from build123d import *

# Parameters (mm, degrees)
SKETCH1_R           = 12.35
BOSS_EXTRUDE1_DEPTH = 68
SKETCH2_R           = 3.55
BOSS_EXTRUDE2_DEPTH = 3
SKETCH3_R           = 2
BOSS_EXTRUDE3_DEPTH = 9.7
SKETCH5_W           = 12.75
SKETCH5_H           = 3
BOSS_EXTRUDE4_DEPTH = 14
SKETCH4_R           = 1.5
CUT_EXTRUDE1_DEPTH  = 3


with BuildPart() as part:
    # Sketch1 → Boss-Extrude1 (new body)
    with BuildSketch(Plane(origin=(0, 0, 0), x_dir=(1, 0, 0), z_dir=(0, 1, 0))):
        Circle(SKETCH1_R)
    extrude(amount=BOSS_EXTRUDE1_DEPTH)

    # Sketch2 → Boss-Extrude2 (add)
    with BuildSketch(Plane(origin=(0, 68, 0), x_dir=(1, 0, 0), z_dir=(0, 1, 0))):
        Circle(SKETCH2_R)
    extrude(amount=BOSS_EXTRUDE2_DEPTH)

    # Sketch3 → Boss-Extrude3 (add)
    with BuildSketch(Plane(origin=(0, 71, 0), x_dir=(1, 0, 0), z_dir=(0, 1, 0))):
        Circle(SKETCH3_R)
    extrude(amount=BOSS_EXTRUDE3_DEPTH)

    # Sketch5 → Boss-Extrude4 (add)
    with BuildSketch(Plane(origin=(0, 0, 0), x_dir=(0, 0, -1), z_dir=(1, 0, 0))):
        with Locations((0, 11.5)):
            Rectangle(SKETCH5_W, SKETCH5_H)
    extrude(amount=BOSS_EXTRUDE4_DEPTH)

    # Sketch4 → Cut-Extrude1 (cut)
    with BuildSketch(Plane(origin=(0, 68, 0), x_dir=(1, 0, 0), z_dir=(0, 1, 0))):
        with Locations((0, 8.5)):
            Circle(SKETCH4_R)
        with Locations((0, -8.5)):
            Circle(SKETCH4_R)
    extrude(amount=-CUT_EXTRUDE1_DEPTH, mode=Mode.SUBTRACT)


solid = part.part
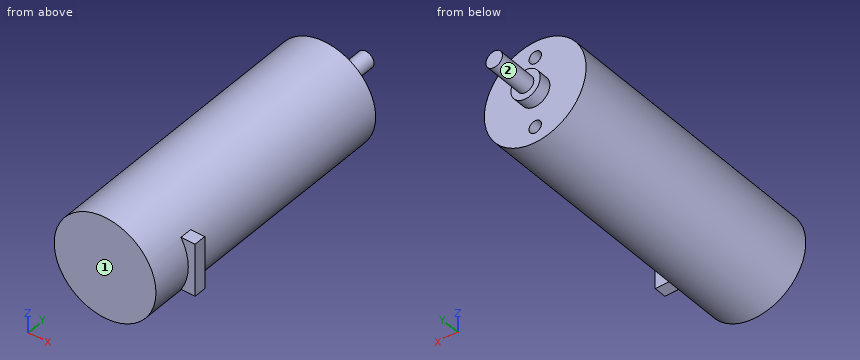
Source: CAD feature listing. Evaluate the final solid. Frame: model axes, mm. Face numbers are marked on the shaded views. A direction names the side the tool comes from. Give positions to 0.01 mm unless a question says otherwise; leave off trailing zeros. Write each loop counter-clockwise with the first axis right and the second up, starting at its lowest first coordinate (ties: lowest second). Pieces come first, ordered by that corner, then holes. Notation, with made-up numbers: (41.25, -34) - (85.25, -34) arc R31 cw to (85.25, -3) - close; hole circle Ø11 at (15.5, -36.5). An arc over 180 degrees is marked (long way). Write item = value, one per line. Start each with the question number.
Q1. Cut plane B-B, the plane z = 0. Return loops of the section in (x, y).
Q2. Reachability of the marked faces 1 and 2 from +Z, -Z, +X, -X, +Y, -Y: full face, straight path, thin tool, end or side. Return the list, or none.
Q3. Cut plane C-C, the plane y = 72. Return loops of the section in (x, z).
Q4. Material intervals for probe 1 along Z at (x, y) = (0, 66); probe 2 along Z at (x, y) = (7.25, 38.5); probe 3 along Y at (x, z) = (5, -7), sorted ascending.
Q5. Pin query (flat end, axial travel): pin 1 Ø2.5 at (x, y) = (12.5, 12) entering from +Z (3 decimals); pin 2 Ø1.5 at (y, z) = (67.5, -4) entering from +X; pin 3 Ø0.9 at (x, y) = (12, 11.5) entering from -Z (3 decimals). Return the tip coordinate at first contact, or that it passes through.
Q6. Cut plane D-D, the plane z = -8.5. Return loops of the section in (x, y), then the cut area to 3 significant figures.
Q7. Cut plane A-A, the plane x = 0. Return loops of the section in (y, z), then the cut area to 3 significant figures.
Computed values:
q1.outline = (-12.35, 0) - (12.35, 0) - (12.35, 10) - (14, 10) - (14, 13) - (12.35, 13) - (12.35, 68) - (3.55, 68) - (3.55, 71) - (2, 71) - (2, 80.7) - (-2, 80.7) - (-2, 71) - (-3.55, 71) - (-3.55, 68) - (-12.35, 68) - close
q2.face_1 = +Z, -Z, +X, -X, -Y
q2.face_2 = +Y
q3.outline = circle Ø4 at (0, 0)
q4.probe_1 = -12.35 to -10, -7 to 7, 10 to 12.35
q4.probe_2 = -10 to 10
q4.probe_3 = 0 to 68
q5.pin_1 = 6.375
q5.pin_2 = 11.91
q5.pin_3 = -6.375
q6.outline = (-8.96, 0) - (8.96, 0) - (8.96, 68) - (1.5, 68) - (1.5, 65) - (-1.5, 65) - (-1.5, 68) - (-8.96, 68) - close
q6.area = 1,210 mm²
q7.outline = (0, -12.35) - (68, -12.35) - (68, -10) - (65, -10) - (65, -7) - (68, -7) - (68, -3.55) - (71, -3.55) - (71, -2) - (80.7, -2) - (80.7, 2) - (71, 2) - (71, 3.55) - (68, 3.55) - (68, 7) - (65, 7) - (65, 10) - (68, 10) - (68, 12.35) - (0, 12.35) - close
q7.area = 1,720 mm²
